Answer from the drawing. Dimensions are ordinates in mm from the lowest x, y and z of the part. A direction names the side the tool comes from. Give positions to 0.01 mm unless a question says otherwise; leave off trailing zeros. Loops run counter-clockwise (first coordinate to the right, second up) from the corner with the lowest first, then second, coordinate; pieces in that order, holes last.
(1) Determine the mould class of the marked faces 4, 5 and 6 for opening direction Z: pulls with the +Z half, pulls with the -Z half, needs draft (parallel to the pull), parting line crosses it, or undercut.
(2) Each of these flat-tipped pins is pushed along its axis until it touches: P1, Ø5, axis at x = 26, y = 4, coming from the +Z side; P2, Ø12, axis at y = 7.5, z = 10, coming from the -X side; P3, Ø1.5, axis at x = 8, z = 14, coming from the -Y side. Where does it stop, or does it pass through?
(3) Which of the six approach directions +Z, -Z, +X, -X, +Y, -Y give full straight-line access (tool end or side, diameter ignored) to the marked faces 1, 2 and 3?
(4) Find section B-B, the plane y = 5. Write down the section's boundary in (x, z).
(5) Find section D-D, the plane y = 13. Write down the section's boundary in (x, z).
(6) Find section A-A, the plane x = 5. Write down the section's boundary in (y, z), then the cut area to 3 significant figures.
(7) Straight lines are drawn through the part: probe 1 along Y at (x, z) = (25, 0.85); probe 2 along Z at (x, y) = (2.5, 2.75); probe 3 along Y at (x, z) = (8.25, 18.25). For each, find the intervals that lie inside material, in ascending order.
(8) Find section C-C, the plane z = 15. Write down the section's boundary in (x, y), then the cut area to 3 significant figures.
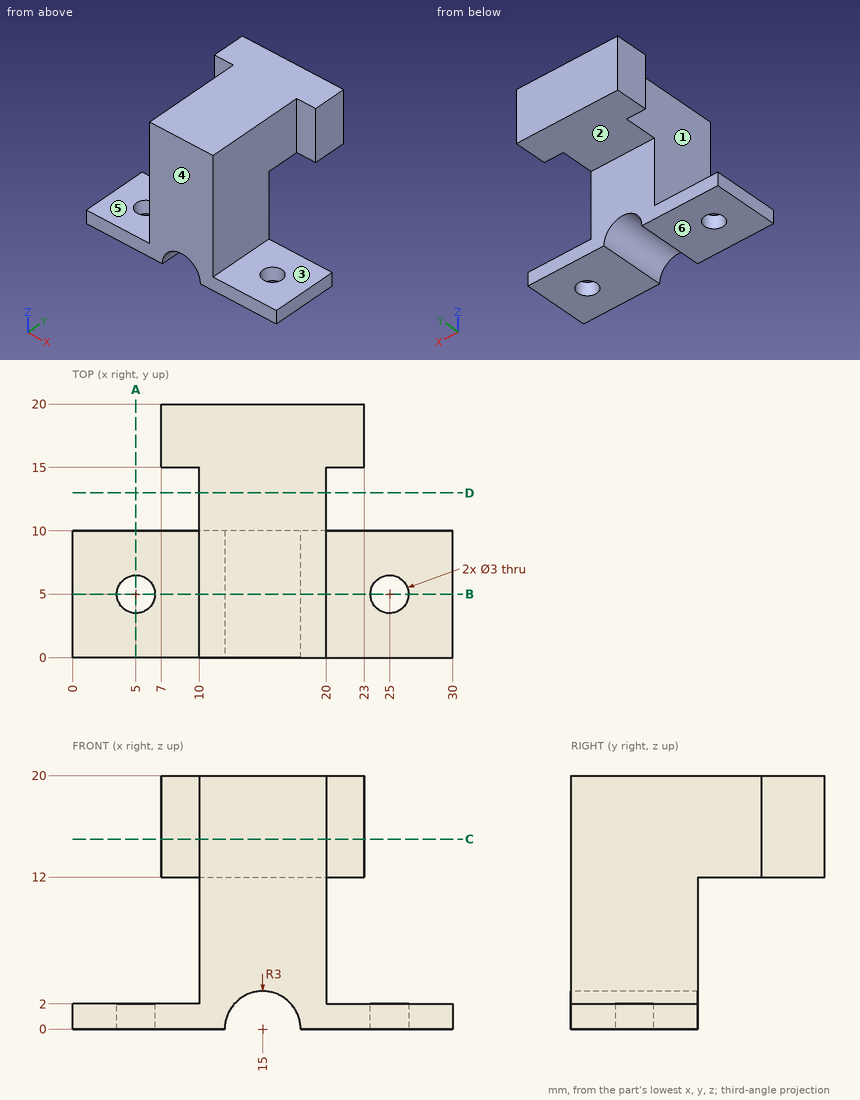
Entries:
1. face 4: needs draft
1. face 5: pulls with the +Z half
1. face 6: pulls with the -Z half
2. P1: stops at z = 2
2. P2: stops at x = 10
2. P3: stops at y = 15
3. face 1: +Z, -X, -Y
3. face 2: -Z, +X, -X, +Y
3. face 3: +Z, +X, +Y, -Y
4. outline: (0, 0) - (3.5, 0) - (3.5, 2) - (0, 2) - close; (6.5, 0) - (12, 0) arc R3 cw to (18, 0) - (23.5, 0) - (23.5, 2) - (20, 2) - (20, 20) - (10, 20) - (10, 2) - (6.5, 2) - close; (26.5, 0) - (30, 0) - (30, 2) - (26.5, 2) - close
5. outline: (10, 12) - (20, 12) - (20, 20) - (10, 20) - close
6. outline: (0, 0) - (3.5, 0) - (3.5, 2) - (0, 2) - close; (6.5, 0) - (10, 0) - (10, 2) - (6.5, 2) - close
6. area: 14.0 mm2
7. probe 1: y = 0 to 3.5, 6.5 to 10
7. probe 2: z = 0 to 2
7. probe 3: y = 15 to 20
8. outline: (7, 15) - (10, 15) - (10, 0) - (20, 0) - (20, 15) - (23, 15) - (23, 20) - (7, 20) - close
8. area: 230 mm2
